Geometry: final body of the model. Coordinates: model frame, mm. Face numbers are marked on the shaded views. A direction names the side the tool comes from. Give positions to 0.01 mm unless a question says otherwise; leave off trailing zeros. Write each loop counter-clockwise with the first axis right and the second up, starting at its lowest first coordinate (ties: lowest second). Pieces come first, ordered by that corner, then holes. Notation, with made-up numbers: (15, 60.5) -> (34, 60.5) arc R14 ccw to (34, 70.5) -> close; hole circle Ø1 at (62, 45). An arc over 180 degrees is marked (long way). Answer as a JSON object with one key per item and string values. Group by question number.
(1) Section query C-C on y = -10.5. Output: boundary loops of the cut face in (x, z), plus the area to 3 significant figures.
(2) Section query D-D on z = 0. Output: boundary loops of the cut face in (x, y).
(3) Draft query along Y for the marked faces 5, 6, 7 and 8. Return one class per face: +Y half, -Y half, draft (parallel to the pull), parting line (faces both ways), or undercut.
(4) Section query B-B on x = -59. State how many separate pieces and enclosed holes the cut face has, plus the area to 3 significant figures.
(5) Set-up query: the marked faces 1, 2, 3 and 4. Return all of +Z, -Z, +X, -X, +Y, -Y with unobstructed straight access to the full face (end or side cutting, diameter ignored); none if empty.
(6) Material intervals for probe 1 along X at (y, z) = (-33, 76.5); probe 2 along X at (y, z) = (-12, 87); probe 3 along Z at (x, y) = (-56, -23.5), sorted ascending.
(7) Contact query for flat-ended pins moving along their axis: pin 1 Ø8 at (x, y) = (81, -2.5) entering from +Z; pin 2 Ø8 at (y, z) = (23, -44.5) entering from +X; pin 3 Ø10 at (y, z) = (-10.5, 39.5) entering from -X. Output: stop coordinate, or through.
(8) Section query A-A on x = 81. Output: boundary loops of the cut face in (y, z) (3 decimals).
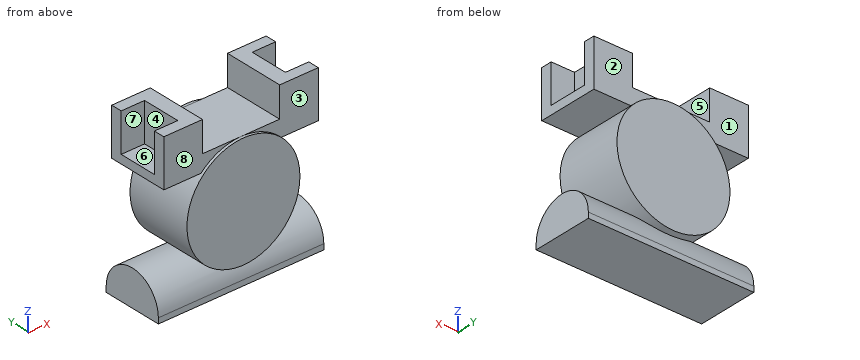
from build123d import *

# Parameters (mm, degrees)
F0_R     = 65.024
F1_DEPTH = 38.1
F3_DEPTH = 95.25
F4_W     = 44.45
F4_H     = 35.052
F5_DEPTH = 34.925
F6_W     = 57.531
F6_H     = 44.45
F6_W_2   = 26.924
F6_H_2   = 22.225
F7_DEPTH = 44.45


with BuildPart() as f1:
    # F0 (on Front) → F1 (new body, symmetric)
    with BuildSketch(Plane.XZ):
        Circle(F0_R)
    extrude(amount=F1_DEPTH, both=True)

    # F2 (on Right) → F3 (join, symmetric)
    with BuildSketch(Plane.YZ):
        with BuildLine():
            Line((34.925, -88.9), (34.925, -82.55))
            ThreePointArc((34.925, -82.55), (24.6957043329, -57.8542956671), (0, -47.625))
            ThreePointArc((0, -47.625), (-24.6957043329, -57.8542956671), (-34.925, -82.55))
            Line((-34.925, -82.55), (-34.925, -88.9))
            Line((-34.925, -88.9), (34.925, -88.9))
        make_face()
    extrude(amount=F3_DEPTH, both=True)

    # F4 (on Front) → F5 (join, symmetric)
    with BuildSketch(Plane.XZ):
        Polygon((-88.9, 45.72), (0, 45.72), (0, 65.024), (-44.45, 65.024), (-44.45, 100.076), (-88.9, 100.076), align=None)
        with Locations((66.675, 82.55)):
            Rectangle(F4_W, F4_H)
        Polygon((0, 65.024), (0, 45.72), (88.9, 45.72), (88.9, 65.024), (44.45, 65.024), align=None)
    extrude(amount=F5_DEPTH, both=True)

    # F6 (on face) → F7 (cut)
    with BuildSketch(Plane.XY.offset(100.076)):
        with Locations((-90.7415, 0)):
            Rectangle(F6_W, F6_H)
        with Locations((75.438, -11.1125)):
            Rectangle(F6_W_2, F6_H_2)
        with Locations((75.438, 11.1125)):
            Rectangle(F6_W_2, F6_H_2)
    extrude(amount=-F7_DEPTH, mode=Mode.SUBTRACT)


solid = f1.part
Answer list:
{
 "1": {"outline": "(-95.25, -88.9) -> (95.25, -88.9) -> (95.25, -49.24) -> (42.47, -49.24) arc R65.02 ccw to (46.24, 45.72) -> (88.9, 45.72) -> (88.9, 55.63) -> (61.98, 55.63) -> (61.98, 100.08) -> (44.45, 100.08) -> (44.45, 65.02) -> (-44.45, 65.02) -> (-44.45, 100.08) -> (-61.98, 100.08) -> (-61.98, 55.63) -> (-88.9, 55.63) -> (-88.9, 45.72) -> (-46.24, 45.72) arc R65.02 ccw to (-42.47, -49.24) -> (-95.25, -49.24) -> close", "area": "22,800 mm2"},
 "2": {"outline": "(-65.02, -38.1) -> (65.02, -38.1) -> (65.02, 38.1) -> (-65.02, 38.1) -> close"},
 "3": {"face 5": "draft", "face 6": "undercut", "face 7": "undercut", "face 8": "-Y half"},
 "4": {"separate pieces": "3", "enclosed holes": "0", "area": "10,300 mm2"},
 "5": {"face 1": "+Z, -X, +Y", "face 2": "+Z, +X, +Y", "face 3": "+Z, +X, -Y", "face 4": "+Z, -X"},
 "6": {"probe 1": "-88.9 to -44.45, 44.45 to 88.9", "probe 2": "-61.98 to -44.45, 44.45 to 61.98", "probe 3": "-88.9 to -56.71, -33.05 to 33.05, 45.72 to 100.08"},
 "7": {"pin 1": "z = 55.63", "pin 2": "x = 50.87", "pin 3": "x = -55.12"},
 "8": {"outline": "(-34.925, -88.9) -> (34.925, -88.9) -> (34.925, -82.55) arc R34.925 ccw to (-34.925, -82.55) -> close; (-34.925, 45.72) -> (34.925, 45.72) -> (34.925, 100.076) -> (22.225, 100.076) -> (22.225, 55.626) -> (-22.225, 55.626) -> (-22.225, 100.076) -> (-34.925, 100.076) -> close"}
}
